Source: CAD feature listing. Evaluate the final solid. Frame: model axes, mm. A direction names the side the tool comes from. Coordinates: 2 decimals unless noted, no trailing zeros. Order: outer loops, then holes, each group sorted by start corner. A loop starts at its lowest first (then second) coordinate and runs counter-clockwise, first axis right, second up.
Item 1: Contact query for flat-ended pins moving along their axis: P1, Ø1.4, axis at x = 53, y = 2, coming from the +Z side; P2, Ø4, axis at x = 2.1, z = 3.75, coming from the +Y side; P3, Ø0.8, axis at y = 1, z = -56.5, coming from the +X side; P4, Ø1.4, axis at x = 20.5, y = 1, coming from the -Z side. Output: stop coordinate, or through.
Item 2: Section C-C on z = -80.5. Return the cut outline in (x, y).
Item 3: Section B-B on x = 13. Return the cut outline in (y, z).
Item 4: Section D-D on y = 1.1. State how many separate pieces and enclosed holes the cut face has, then the cut area to 3 significant figures.
Item 5: Ray query, line 1 (Z direction, x = 2.1, y = 1.25); line 2 (Z direction, x = 32.5, y = 0.35); line 3 (X direction, y = 1.05, z = -58.5). Return the intervals inside material, ascending.
Item 6: Section A-A on x = 62.9. Return the cut outline in (y, z).
Item 7: Reachability of faces 1 (the flat face through (33, 1, -89.148)), 2 (the flat face through (42.63, 1.42, 4.37)), 3 (the flat face through (65, 1, -41)) from +Z, -Z, +X, -X, +Y, -Y: full face, straight path, thin tool, end or side. Return the list, or none.
Item 8: Mould query, pull axis Z, two halves, no side actions, for faces 4 (the flat face through (32, 2.8, -42)), 5 (the cylindrical face through (62.63, 1.38, -89.13)), 6 (the flat face through (46, 1, 5.852)), 7 (the cylindrical face through (3.23, 1.38, 1.98)). Classes: released by +Z, released by -Z, zero draft, split by the parting line, or undercut.
from build123d import *

# Parameters (mm, degrees)
SKETCH1_R           = 2.1
BOSS_EXTRUDE1_DEPTH = 2.8
CUT_EXTRUDE1_REACH  = 4.8
FILLET1_R           = 0.5


with BuildPart() as part:
    # Sketch1 → Boss-Extrude1 (new body)
    with BuildSketch(Plane(origin=(0, 0, 0), x_dir=(1, 0, 0), z_dir=(0, 1, 0))):
        with BuildLine():
            Line((0, 83.295334784), (0, 0))
            ThreePointArc((0, 0), (-0.940559159, -6.792891767), (5.852332608, -5.852332608))
            Line((5.852332608, -5.852332608), (59.147667392, -5.852332608))
            ThreePointArc((59.147667392, -5.852332608), (65.940559159, -6.792891767), (65, 0))
            Line((65, 0), (65, 83.295334784))
            ThreePointArc((65, 83.295334784), (65.940559159, 90.088226551), (59.147667392, 89.147667392))
            Line((59.147667392, 89.147667392), (5.852332608, 89.147667392))
            ThreePointArc((5.852332608, 89.147667392), (-0.940559159, 90.088226551), (0, 83.295334784))
        make_face()
        with Locations((2.1, 87.047667392)):
            Circle(SKETCH1_R, mode=Mode.SUBTRACT)
        with Locations((2.1, -3.752332608)):
            Circle(SKETCH1_R, mode=Mode.SUBTRACT)
        with Locations((62.9, -3.752332608)):
            Circle(SKETCH1_R, mode=Mode.SUBTRACT)
        with Locations((62.9, 87.047667392)):
            Circle(SKETCH1_R, mode=Mode.SUBTRACT)
    extrude(amount=BOSS_EXTRUDE1_DEPTH)

    # Sketch2 → Cut-Extrude1 (cut, up to next)
    with BuildSketch(Plane(origin=(0, 2.8, 0), x_dir=(1, 0, 0), z_dir=(0, 1, 0)), mode=Mode.PRIVATE) as cut_extrude1_sk1:
        Polygon((22.9, -2.852332608), (21.852379604, -5.852332608), (43.147620396, -5.852332608), (42.1, -2.852332608), align=None)
    cut_extrude1_tool1 = extrude(cut_extrude1_sk1.sketch, amount=-CUT_EXTRUDE1_REACH, mode=Mode.PRIVATE) & part.part
    add(cut_extrude1_tool1.solids().sort_by_distance((32.5, 2.8, 4.378203))[0], mode=Mode.SUBTRACT)
    # Sketch2 → Cut-Extrude1 (cut, up to next)
    with BuildSketch(Plane(origin=(0, 2.8, 0), x_dir=(1, 0, 0), z_dir=(0, 1, 0)), mode=Mode.PRIVATE) as cut_extrude1_sk2:
        with BuildLine():
            Line((15.852379604, -5.852332608), (14.804759208, -2.852332608))
            Line((14.804759208, -2.852332608), (6.304759208, -2.852332608))
            ThreePointArc((6.304759208, -2.852332608), (6.351920453, -4.393559913), (5.852332608, -5.852332608))
            Line((5.852332608, -5.852332608), (15.852379604, -5.852332608))
        make_face()
    cut_extrude1_tool2 = extrude(cut_extrude1_sk2.sketch, amount=-CUT_EXTRUDE1_REACH, mode=Mode.PRIVATE) & part.part
    add(cut_extrude1_tool2.solids().sort_by_distance((10.801148, 2.8, 4.393371))[0], mode=Mode.SUBTRACT)
    # Sketch2 → Cut-Extrude1 (cut, up to next)
    with BuildSketch(Plane(origin=(0, 2.8, 0), x_dir=(1, 0, 0), z_dir=(0, 1, 0)), mode=Mode.PRIVATE) as cut_extrude1_sk3:
        with BuildLine():
            Line((59.147667392, -5.852332608), (49.147620396, -5.852332608))
            Line((49.147620396, -5.852332608), (50.195240792, -2.852332608))
            Line((50.195240792, -2.852332608), (58.695240792, -2.852332608))
            ThreePointArc((58.695240792, -2.852332608), (58.648079547, -4.393559913), (59.147667392, -5.852332608))
        make_face()
    cut_extrude1_tool3 = extrude(cut_extrude1_sk3.sketch, amount=-CUT_EXTRUDE1_REACH, mode=Mode.PRIVATE) & part.part
    add(cut_extrude1_tool3.solids().sort_by_distance((54.198852, 2.8, 4.393371))[0], mode=Mode.SUBTRACT)

    # Fillet1
    fillet1_edges = [part.edges().sort_by_distance(p)[0] for p in [
        (5.852332608, 1.4, -89.147667392),
        (59.147667392, 1.4, -89.147667392),
        (65, 1.4, -83.295334784),
        (65, 1.4, 0),
        (0, 1.4, 0),
        (0, 1.4, -83.295334784),
        (58.695240792, 1.4, 2.852332608),
        (49.147620396, 1.4, 5.852332608),
        (50.195240792, 1.4, 2.852332608),
        (15.852379604, 1.4, 5.852332608),
        (6.304759208, 1.4, 2.852332608),
        (14.804759208, 1.4, 2.852332608),
        (22.9, 1.4, 2.852332608),
        (42.1, 1.4, 2.852332608),
        (43.147620396, 1.4, 5.852332608),
        (21.852379604, 1.4, 5.852332608),
    ]]
    fillet(fillet1_edges, radius=FILLET1_R)


solid = part.part
Answer list:
1. P1: stops at z = 2.85
1. P2: passes through
1. P3: stops at x = 65
1. P4: stops at z = -89.15
2. outline: (0, 0) - (65, 0) - (65, 2.8) - (0, 2.8) - close
3. outline: (0, -89.15) - (2.8, -89.15) - (2.8, 2.85) - (0, 2.85) - close
4. separate pieces: 1
4. enclosed holes: 4
4. area: 6,090 mm2
5. line 1: z = -91.35 to -89.15, -84.95 to 1.65, 5.85 to 8.05
5. line 2: z = -89.15 to 2.85
5. line 3: x = 0 to 65
6. outline: (0, -91.35) - (2.8, -91.35) - (2.8, -89.15) - (0, -89.15) - close; (0, -84.95) - (2.8, -84.95) - (2.8, 1.65) - (0, 1.65) - close; (0, 5.85) - (2.8, 5.85) - (2.8, 8.05) - (0, 8.05) - close
7. face 1: -Z, +Y, -Y
7. face 2: +Z, +Y, -Y
7. face 3: +X, +Y, -Y
8. face 4: zero draft
8. face 5: undercut
8. face 6: released by +Z
8. face 7: undercut
